from build123d import *

# Parameters (mm, degrees)
SKETCH4_W                      = 3
SKETCH4_H                      = 1
SKETCH5_W                      = 47.328638264
SKETCH5_H                      = 14
CUT_EXTRUDE1_DEPTH             = 77
F_1_2_0_51181102_DOWEL_HOLE1_D = 12.999999908
CHAMFER1_SIZE                  = 2


with BuildPart() as part:
    # Sketch2 → Revolve1 (revolve)
    with BuildSketch(Plane.XY, mode=Mode.PRIVATE) as revolve1_sk:
        Polygon((-63.5, 0), (-63.5, 17.5), (-28.5, 17.5), (-28.5, 27), (0.5, 27), (0.5, 17.5), (63.5, 17.5), (63.5, 0), align=None)
    revolve(revolve1_sk.sketch.rotate(Axis((-63.5, 0, 0), (1, 0, 0)), 90), axis=Axis((-63.5, 0, 0), (1, 0, 0)))

    # Sketch4 → Cut-Revolve1 (revolve, cut)
    with BuildSketch(Plane.XY, mode=Mode.PRIVATE) as cut_revolve1_sk:
        with Locations((-30, 17)):
            Rectangle(SKETCH4_W, SKETCH4_H)
    revolve(cut_revolve1_sk.sketch.rotate(Axis((-63.5, 0, 0), (1, 0, 0)), 90), axis=Axis((-63.5, 0, 0), (1, 0, 0)), mode=Mode.SUBTRACT)

    # Sketch5 → Cut-Extrude1 (cut)
    with BuildSketch(Plane(origin=(63.5, 0, 0), x_dir=(0, 0, -1), z_dir=(1, 0, 0))):
        with Locations((0, 20)):
            Rectangle(SKETCH5_W, SKETCH5_H)
    extrude(amount=-CUT_EXTRUDE1_DEPTH, mode=Mode.SUBTRACT)

    # 1/2 (0.51181102) Dowel Hole1 (through all)
    with Locations(Plane(origin=(0, 13, 0), x_dir=(1, 0, 0), z_dir=(0, 1, 0))):
        with Locations((41.5, 0)):
            Hole(F_1_2_0_51181102_DOWEL_HOLE1_D / 2)

    # Chamfer1
    chamfer1_edges = [part.edges().sort_by_distance(p)[0] for p in [
        (63.5, -17.5, 0),
        (-63.5, 0, -17.5),
    ]]
    chamfer(chamfer1_edges, length=CHAMFER1_SIZE)


solid = part.part
Read the model definition and answer for the solid it produces. Units are mm, in the model's axes. A direction names the side the tool comes from. Give positions to 0.01 mm unless a question says otherwise; leave off trailing zeros. Loops run counter-clockwise (first coordinate to the right, second up) from the corner with the lowest first, then second, coordinate; pieces in that order, holes last. Notation, with made-up numbers: (70.25, 16.25) -> (102.25, 16.25) arc R16 ccw to (102.25, 26.25) -> close; hole circle Ø11 at (-25.5, -9). An arc over 180 degrees is marked (long way). Use a Markdown table: item, result.
Q1. Find the intervals of material crossed by line 1 along Z through (x, y) = (-33, 1); line 2 along X through (y, z) = (-5, -1.5); line 3 along Z through (x, y) = (41, -10), in increasing order.
Solved:
| item | result |
|---|---|
| line 1 | z = -17.47 to 17.47 |
| line 2 | x = -63.5 to 35.18, 47.82 to 63.5 |
| line 3 | z = -14.36 to -6.48, 6.48 to 14.36 |
Q2. Section C-C, the plane x = 41.5 is taken. Determine the outline of the cut face in (y, z).
Solved:
| item | result |
|---|---|
| outline | (-16.25, -6.5) arc R17.5 ccw to (13, -11.72) -> (13, -6.5) -> close; (-16.25, 6.5) -> (13, 6.5) -> (13, 11.72) arc R17.5 ccw to start |
Q3. Each of these flat-tipped pins is pushed along its axis until it touches: pin 1 (1.5 mm diameter, centred on y = 14.5, z = 14.5, fed in from -X); pin 2 (8 mm diameter, centred on y = -12.5, z = 21.5, fed in from +X); pin 3 (4 mm diameter, centred on x = 50, z = 1, fed in from +Y); pin 4 (11.5 mm diameter, centred on x = 41.5, z = 0, fed in from +Y). Where does it stop, or does it pass through?
Solved:
| item | result |
|---|---|
| pin 1 | stops at x = -28.5 |
| pin 2 | stops at x = 0.5 |
| pin 3 | stops at y = 13 |
| pin 4 | passes through |
Q4. A tool of negligible diameter and unlimited length cuts with its end or side. For faces 4 (the face through (-46.29, 17.084, -3.794)), 5 (the face through (31.43, -17.49, 0.59)), 6 (the face through (17, 13, 0)), 7 (the face through (-31.5, -5, 16)), from which of +Z, -Z, +X, -X, +Y, -Y can it reach the whole face along a straight path? Write none if from no direction.
Solved:
| item | result |
|---|---|
| face 4 | -X |
| face 5 | +X |
| face 6 | +Z, -Z, +X, +Y |
| face 7 | none |
Q5. Determine the mould class of faces 1 (the face through (-29.979, -4.956, 15.738)), 2 (the face through (63.5, -1, 0)), 3 (the face through (-63.5, 0, 0)) for opening direction X: pulls with the +X half, pulls with the -X half, needs draft (parallel to the pull), parting line crosses it, or undercut.
Solved:
| item | result |
|---|---|
| face 1 | undercut |
| face 2 | pulls with the +X half |
| face 3 | pulls with the -X half |
Q6. Section A-A, the plane z = 0 is taken. Determine the outline of the cut face in (x, y), then the cut area to 3 significant figures.
Solved:
| item | result |
|---|---|
| outline | (-63.5, -15.5) -> (-61.5, -17.5) -> (-31.5, -17.5) -> (-31.5, -16.5) -> (-28.5, -16.5) -> (-28.5, -27) -> (0.5, -27) -> (0.5, -17.5) -> (35, -17.5) -> (35, 13) -> (-13.5, 13) -> (-13.5, 27) -> (-28.5, 27) -> (-28.5, 16.5) -> (-31.5, 16.5) -> (-31.5, 17.5) -> (-61.5, 17.5) -> (-63.5, 15.5) -> close; (48, -17.5) -> (61.5, -17.5) -> (63.5, -15.5) -> (63.5, 13) -> (48, 13) -> close |
| area | 4,110 mm^2 |
Q7. Section B-B, the plane x = -17 is taken. Determine the outline of the cut face in (y, z).
Solved:
| item | result |
|---|---|
| outline | circle Ø54 at (0, 0) |
Q8. Section D-D, the plane x = -43 is taken. Determine the outline of the cut face in (y, z).
Solved:
| item | result |
|---|---|
| outline | circle Ø35 at (0, 0) |
